Autodesk Inventor part; units mm, degrees
ref_plane "Work Plane1" through (0, 0, -6) normal (0, 0, 1) x (1, 0, 0)
ref_plane "YZ Plane" through (0, 0, 0) normal (1, 0, 0) x (0, 1, 0)
ref_plane "XZ Plane" through (0, 0, 0) normal (0, 1, 0) x (-1, 0, 0)
sketch "Sketch1" plane through (0, 0, 0) normal (0, 0, 1) x (1, 0, 0)
  circle A0 centre (0, 0) radius 7
  circle A1 centre (0, 65) radius 3
  line L0 (-57.25, -10) -> (57.25, -10)
  line L1 (57.25, -10) -> (57.25, 90)
  line L2 (57.25, 90) -> (-57.25, 90)
  line L3 (-57.25, 90) -> (-57.25, -10)
  line L4 (0, 65) -> (0, 0) construction
  point P0 (0, 32.5)
  point P1 (-57.25, 40)
  point P2 (0, 90)
  dimension "d0" = 14
  dimension "d1" = 6
  dimension "d2" = 65
  dimension "d3" = 114.5
  dimension "d7" = 25
  dimension "d8" = 10
extrude "Extrusion1" add sketch "Sketch1" along normal blind 10
sketch "Sketch2" plane through (-57.25, -10, 0) normal (0, -1, 0) x (1, 0, 0)
  line L0 (0, 10) -> (114.5, 10)
  line L1 (0, 10) -> (114.5, 10)
  line L2 (114.5, 10) -> (114.5, -35)
  line L3 (114.5, -35) -> (0, -35)
  line L4 (0, -35) -> (0, 10)
  point P0 (57.25, 0)
  point P1 (114.5, 0)
  dimension "d10" = 45
extrude "Extrusion2" add sketch "Sketch2" along normal blind 10
sketch "Sketch3" plane through (0, 0, 0) normal (0, 0, -1) x (-1, 0, 0)
  circle A0 centre (0, 0) radius 22.5 construction
  circle A1 centre (0, 0) radius 7
  line L0 (-22.5, 0) -> (-22.5, -10)
  line L1 (57.25, -10) -> (-57.25, -10) construction
  line L2 (22.5, 0) -> (22.5, -10)
  arc A2 (22.5, 0) -> (-22.5, 0) centre (0, 0) ccw
  line L3 (-22.5, -10) -> (22.5, -10)
  dimension "d13" = 45
extrude "Extrusion3" add sketch "Sketch3" along normal blind 35
sketch "Sketch4" plane through (-57.25, 90, 0) normal (-1, 0, 0) x (0, 0, 1)
  line L0 (-35, -100) -> (0, -100)
  line L1 (-35, -100) -> (0, 0)
  line L2 (0, 0) -> (10, 0)
  line L3 (0, 0) -> (10, 0)
  line L4 (10, 0) -> (10, -110)
  line L5 (10, 0) -> (10, -110)
  line L6 (10, -110) -> (-35, -110)
  line L7 (10, -110) -> (-35, -110)
  line L8 (-35, -100) -> (-35, -110)
  line L9 (-35, -110) -> (-35, -100)
extrude "Extrusion4" add sketch "Sketch4" against normal blind 10
sketch "Sketch5" plane through (57.25, 90, 10) normal (1, 0, 0) x (0, 0, -1)
  line L0 (45, -100) -> (10, 0)
  line L1 (10, -100) -> (10, 0)
  line L2 (45, -100) -> (10, -100)
  point P0 (0, -110)
extrude "Extrusion5" add sketch "Sketch5" against normal blind 10
sketch "Sketch6" plane through (0, 0, 0) normal (0, 0, -1) x (-1, 0, 0)
  circle A0 centre (0, 65) radius 3
  circle A1 centre (8.75, 65) radius 2
  circle A2 centre (-8.75, 65) radius 2
  line L0 (-8.75, 65) -> (8.75, 65) construction
  point P0 (0, 0)
  point P1 (0, 65)
  dimension "d20" = 4
  dimension "d21" = 4
  dimension "d22" = 17.5
extrude "Extrusion6" cut sketch "Sketch6" against normal through all contours A1 | A2
sketch "Sketch9" plane through (0, 0, 0) normal (0, 0, -1) x (-1, 0, 0)
  circle A0 centre (0, 65) radius 3
  circle A1 centre (0, 65) radius 15
  point P0 (0, 0)
  dimension "d28" = 30
extrude "Extrusion8" cut sketch "Sketch9" against normal blind 5
sketch "Sketch10" plane through (-57.25, -10, 0) normal (0, 1, 0) x (1, 0, 0)
  circle A0 centre (83.5, 20) radius 2
  line L0 (0, 0) -> (0, 35)
  circle A1 centre (31, 20) radius 2
  line L1 (34.75, 35) -> (79.75, 35)
  line L2 (34.75, 35) -> (79.75, 35)
  line L3 (83.5, 20) -> (31, 20)
  line L4 (79.75, 35) -> (34.75, 35)
  point P0 (57.25, 0)
  point P1 (114.5, 35)
  point P2 (57.25, 20)
  point P3 (57.25, 35)
  dimension "d31" = 4
  dimension "d33" = 4
  dimension "d55" = 15
  dimension "d57" = 52.5
extrude "Extrusion9" cut sketch "Sketch10" against normal through all
sketch "Sketch11" plane through (0, 0, -35) normal (0, 0, -1) x (-1, 0, 0)
  line L0 (57.25, -20) -> (-57.25, -20)
  line L1 (-57.25, -20) -> (-57.25, -39)
  line L2 (-57.25, -39) -> (57.25, -39)
  line L3 (57.25, -39) -> (57.25, -20)
  point P0 (0, 0)
  point P1 (57.25, -20)
  point P2 (-57.25, -20)
  point P3 (0, -20)
  dimension "d36" = 19
extrude "Extrusion10" add sketch "Sketch11" against normal blind 8.5
sketch "Sketch12" plane through (0, 0, -35) normal (0, 0, -1) x (-1, 0, 0)
  circle A0 centre (-35, -29) radius 2
  circle A1 centre (35, -29) radius 2
  line L0 (-35, -29) -> (35, -29) construction
  line L1 (-57.25, -39) -> (57.25, -39)
  point P0 (0, 0)
  point P1 (0, -29)
  point P2 (0, -39)
  dimension "d39" = 4
  dimension "d40" = 4
  dimension "d41" = 70
  dimension "d42" = 10
extrude "Extrusion11" cut sketch "Sketch12" against normal through all
ref_plane "Work Plane1" through (0, 0, -6) normal (0, 0, 1) x (1, 0, 0)
sketch "Sketch14" plane through (0, 0, -6) normal (0, 0, 1) x (1, 0, 0)
  circle A0 centre (35, -29) radius 2
  circle A1 centre (-35, -29) radius 2
  line L0 (-57.25, -20) -> (57.25, -20)
  line L1 (-57.25, -20) -> (-57.25, -39)
  line L2 (-57.25, -39) -> (57.25, -39)
  line L3 (57.25, -39) -> (57.25, -20)
  point P0 (0, 0)
extrude "Extrusion12" add sketch "Sketch14" along normal blind 10 contours A0 | A1 | L0 L3 L2 L1
sketch "Sketch15" plane through (0, 0, 4) normal (0, 0, 1) x (1, 0, 0)
  circle A0 centre (0, -29) radius 2
  line L0 (-57.25, -39) -> (57.25, -39)
  point P0 (0, 0)
  point P1 (0, -39)
  dimension "d48" = 4
  dimension "d49" = 10
extrude "Extrusion13" cut sketch "Sketch15" against normal blind 10
sketch "Sketch16" plane through (0, 0, 4) normal (0, 0, 1) x (1, 0, 0)
  circle A0 centre (0, -29) radius 2
  line L0 (-57.25, -20) -> (57.25, -20)
  line L1 (-57.25, -20) -> (-57.25, -39)
  line L2 (-57.25, -39) -> (57.25, -39)
  line L3 (57.25, -39) -> (57.25, -20)
  circle A1 centre (0, -29) radius 2
  circle A2 centre (0, -29) radius 7.5
  point P0 (0, 0)
  dimension "d52" = 15
extrude "Extrusion14" add sketch "Sketch16" along normal blind 6 contours L0 L3 L2 L1
sketch "Sketch17" plane through (-57.25, -10, 0) normal (0, 1, 0) x (1, 0, 0)
  line L0 (114.5, 6) -> (0, 6)
  line L1 (0, 6) -> (0, 26.5)
  line L2 (0, 26.5) -> (114.5, 26.5)
  line L3 (114.5, 26.5) -> (114.5, 6)
  circle A0 centre (83.5, 20) radius 2
  circle A1 centre (31, 20) radius 2
  line L4 (0, 6) -> (0, 26.5)
  line L5 (0, 26.5) -> (-36.5, -10) construction
  line L6 (0, 26.5) -> (51.6188, 26.5) construction
  line L7 (114.5, -10) -> (0, -10)
  line L8 (0, -10) -> (-36.5, -10) construction
  line L9 (0, 26.5) -> (0, -10)
  line L10 (114.5, 26.5) -> (114.5, 6)
  line L11 (114.5, 26.5) -> (151, -10) construction
  line L12 (114.5, -10) -> (151, -10) construction
  line L13 (114.5, -10) -> (114.5, 26.5)
  line L14 (129.5, 11.5) -> (129.5, -10)
  line L15 (114.5, 26.5) -> (129.5, 11.5)
  line L16 (129.5, -10) -> (114.5, -10)
  line L17 (-15, 11.5) -> (-15, -10)
  line L18 (0, 35) -> (0, 26.5)
  line L19 (0, 26.5) -> (-15, 11.5)
  line L20 (0, -10) -> (-15, -10)
  point P0 (57.25, 0)
  dimension "d58" = 135
  dimension "d60" = 135
  dimension "d65" = 15
  dimension "d66" = 15
extrude "Extrusion15" add sketch "Sketch17" along normal blind 100 contours L3 L15 L14 L16 L13 | L9 L20 L17 L19 L1
sketch "Sketch18" plane through (57.25, 14.2857, -26.5) normal (-1, 0, 0) x (0, 0, 1)
  line L0 (26.5, 75.7143) -> (-8.5, -24.2857) construction
  line L1 (26.5, -24.2857) -> (-8.5, -24.2857) construction
  line L2 (26.5, 75.7143) -> (26.5, -24.2857) construction
  line L3 (-8.5, -24.2857) -> (-8.5, 75.7143)
  line L4 (-8.5, 75.7143) -> (26.5, 75.7143)
  line L5 (-8.5, -24.2857) -> (26.5, 75.7143)
extrude "Extrusion16" cut sketch "Sketch18" along normal through all both and the other way through all
sketch "Sketch19" plane through (-72.25, -10, -11.5) normal (-0.7071, 0, -0.7071) x (-0.7071, 0, 0.7071)
  circle A0 centre (-10.6066, 15) radius 1.5
  line L0 (-21.2132, 0) -> (0, 0)
  point P0 (-42.9567, 10)
  point P1 (-10.6066, 0)
  dimension "d67" = 3
  dimension "d68" = 15
extrude "Extrusion17" cut sketch "Sketch19" against normal through all
sketch "Sketch20" plane through (72.25, -10, -11.5) normal (0.7071, 0, -0.7071) x (-0.7071, 0, -0.7071)
  circle A0 centre (10.6066, 15) radius 1.5
  line L0 (0, 0) -> (21.2132, 0)
  point P0 (42.9567, 10)
  point P1 (10.6066, 0)
  dimension "d71" = 3
  dimension "d72" = 15
extrude "Extrusion18" cut sketch "Sketch20" against normal through all
sketch "Sketch21" plane through (-47.25, 90, 0) normal (0, 1, 0) x (1, 0, 0)
  line L0 (-25, -10) -> (-10, -10)
  line L1 (-25, -10) -> (-19.6967, -4.6967) construction
  line L2 (-25, -10) -> (-17.5, -10) construction
  line L3 (-25, 11.5) -> (-25, -10)
  line L4 (-25, 0.6066) -> (-14.3934, -10)
  line L5 (-25, 0.6066) -> (-25, -10)
  line L6 (-14.3934, -10) -> (-25, -10)
  line L7 (-25, -10) -> (119.5, -10)
  line L8 (119.5, -10) -> (114.1967, -4.6967) construction
  line L9 (119.5, -10) -> (127, -10) construction
  line L10 (108.8934, -10) -> (119.5, 0.6066)
  line L11 (119.5, -10) -> (119.5, 11.5)
  line L12 (108.8934, -10) -> (123.8934, -10) construction
  line L13 (108.8934, -10) -> (119.5, -10)
  line L14 (119.5, -10) -> (119.5, 0.6066)
  point P0 (47.25, 0)
  dimension "d75" = 7.5
  dimension "d76" = 45
  dimension "d77" = 7.5
  dimension "d78" = 135
  dimension "d79" = 45
extrude "Extrusion19" cut sketch "Sketch21" against normal through all
sketch "Sketch22" plane through (0, 0, 10) normal (0, 0, 1) x (1, 0, 0)
  circle A0 centre (0, 0) radius 14.5
  circle A1 centre (0, 0) radius 7
  dimension "d82" = 29
extrude "Extrusion20" cut sketch "Sketch22" against normal blind 8
sketch "Sketch23" plane through (-47.25, -10, -35) normal (0, 0, -1) x (-1, 0, 0)
  circle A0 centre (-47.25, 10) radius 7
  circle A1 centre (-47.25, 10) radius 14.5
  dimension "d85" = 29
extrude "Extrusion21" cut sketch "Sketch23" against normal blind 16.5
sketch "Sketch24" plane through (0, 65, 5) normal (0, 0, -1) x (-1, 0, 0)
  circle A0 centre (0, 0) radius 3
  circle A1 centre (0, 0) radius 4
  point P0 (0, -65)
  dimension "d88" = 8
extrude "Extrusion22" cut sketch "Sketch24" against normal blind 3
sketch "Sketch25" plane through (0, 0, 10) normal (0, 0, 1) x (1, 0, 0)
  circle A0 centre (-8.75, 65) radius 2
  circle A1 centre (8.75, 65) radius 2
  circle A2 centre (8.75, 65) radius 3
  circle A3 centre (-8.75, 65) radius 3
  point P0 (0, 0)
  dimension "d91" = 6
  dimension "d92" = 6
extrude "Extrusion23" cut sketch "Sketch25" against normal blind 2 contours A0 | A1 | A2 | A3
properties part number "WA004" material "ABS Plastic"
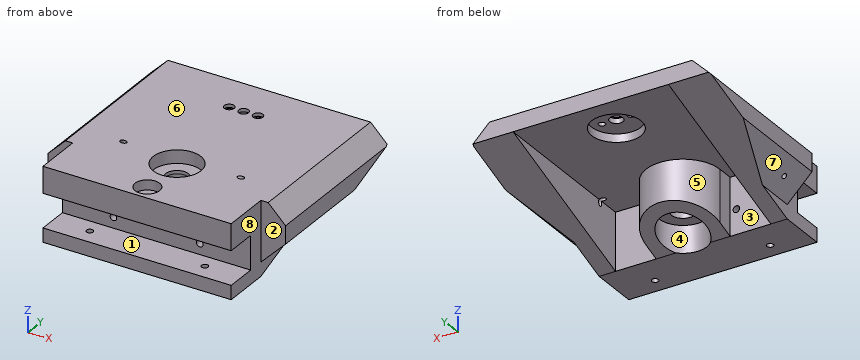
CAD build for the part. Positions are in the model's coordinates, mm. Face numbers are marked on the shaded views. A direction names the side the tool comes from. Round coordinates to 2 decimals unless told otherwise and drop trailing zeros. Write each loop counter-clockwise with the first axis right and the second up, starting at its lowest first coordinate (ties: lowest second). Pieces come first, ordered by that corner, then holes. Notation, with made-up numbers: (-19.75, 48) -> (6.25, 48) arc R34 ccw to (6.25, 79) -> close; hole circle Ø4 at (-32.5, -14.75). An arc over 180 degrees is marked (long way). Answer in a Markdown table with one row per item. Add a question column.
Item 1: Drill centre lines: line 1 (Y direction, x = 0, z = -5); line 2 (Y direction, x = 0, z = 9.5); line 3 (X direction, y = 0, z = -28). Where is each one in solid material? Low to high. Write a range as from..to.
Item 2: Drop flat-ended pins along their axis: pin 1 Ø4.5 at (x, y) = (3, -28) entering from +Z; pin 2 Ø4.5 at (x, z) = (-26.25, -20) entering from +Y; pin 3 Ø3 at (x, y) = (0, -29) entering from +Z. Give the stop position or say it passes through.
Item 3: Mould opens along X. For the marked faces 5, 6, 7 and 8 say: pulls with the +X half, pulls with the -X half, needs draft (parallel to the pull), parting line crosses it, or undercut.
Item 4: Saw through at A-A, the plane x = 26.25. Write the cut outline in (y, z), then the cut area to 3 significant figures.
Item 5: Saw through at B-B, the plane y = 37.5. Write the cut outline in (x, z) (3 decimals).
Item 6: Which spindle directions (+Z, -Z, +X, -X, +Y, -Y) get a long thin tool onto all of the face, cutting with end or side? Do the marked faces 1, 2, 3 and 4. Say none if no direction does.
Item 7: Saw through at C-C, the plane x = 0. Count the separate pieces of the cut face and the enclosed holes in it, then the cut area to 3 significant figures.
Findings below:
| question | item | result |
|---|---|---|
| 1 | line 1 | y = -39..-31, -27..-7, 7..22.5 |
| 1 | line 2 | y = -39..-36.5, -21.5..-14.5, 14.5..62, 68..90 |
| 1 | line 3 | x = -57.25..-47.25, -22.5..-14.5, 14.5..22.5, 47.25..57.25 |
| 2 | pin 1 | stops at z = 4 |
| 2 | pin 2 | stops at y = -10 |
| 2 | pin 3 | stops at z = -26.5 |
| 3 | face 5 | undercut |
| 3 | face 6 | needs draft |
| 3 | face 7 | pulls with the -X half |
| 3 | face 8 | pulls with the +X half |
| 4 | outline | (-39, -35) -> (-10, -35) -> (-10, -22) -> (-20, -22) -> (-20, -26.5) -> (-39, -26.5) -> close; (-39, -6) -> (-20, -6) -> (-20, -18) -> (-10, -18) -> (-10, 0) -> (90, 0) -> (90, 10) -> (-39, 10) -> close |
| 4 | area | 1,880 mm^2 |
| 5 | outline | (-72.25, -11.5) -> (-65.375, -18.375) -> (-47.25, -18.375) -> (-47.25, 0) -> (47.25, 0) -> (47.25, -18.375) -> (65.375, -18.375) -> (72.25, -11.5) -> (72.25, -0.607) -> (61.643, 10) -> (-61.643, 10) -> (-72.25, -0.607) -> close |
| 6 | face 1 | +X, -X, -Y |
| 6 | face 2 | +Z, -Z, +X, -Y |
| 6 | face 3 | -Z, +Y |
| 6 | face 4 | -Z |
| 7 | separate pieces | 4 |
| 7 | enclosed holes | 0 |
| 7 | area | 1,660 mm^2 |
